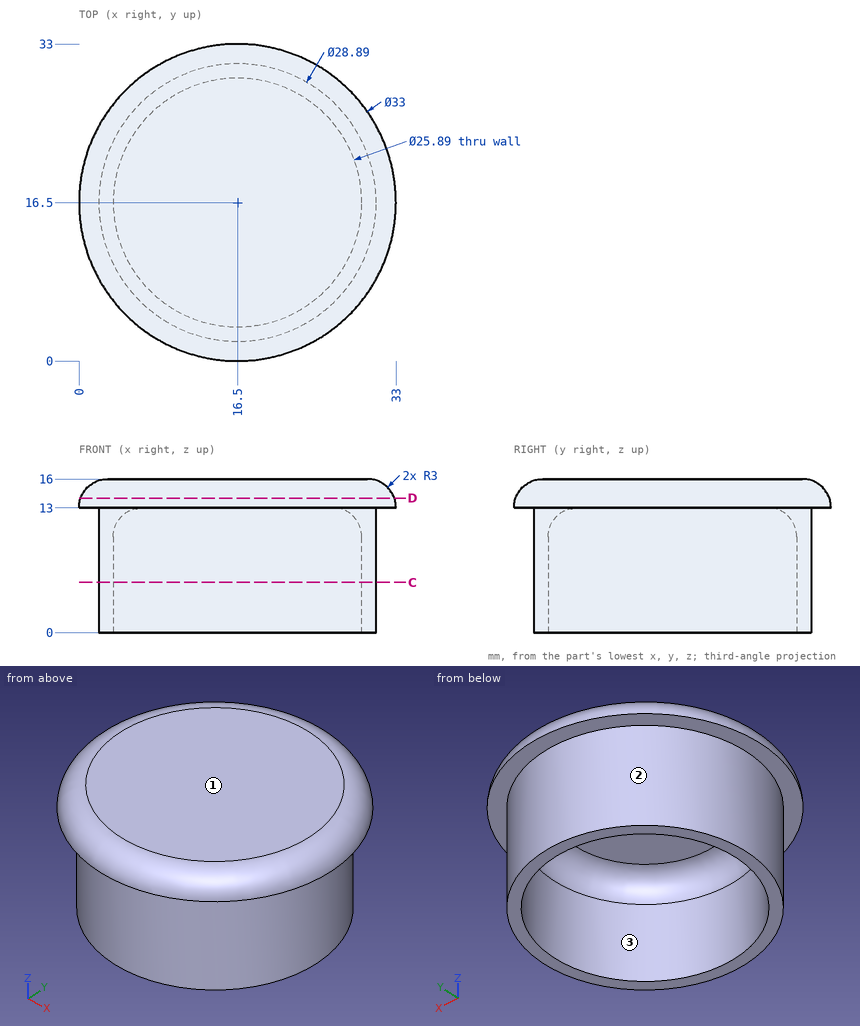
Here's the drawing with two shaded views (mm, measured from the low corner). I have some questions. Round coordinates to 2 decimals unless told otherwise and drop trailing zeros. Write each loop counter-clockwise with the first axis right and the second up, starting at its lowest first coordinate (ties: lowest second). Pieces come first, ordered by that corner, then holes.
(1) If I drill on probe 1 along Y at (x, z) = (16.5, 6) (3 decimals); probe 2 along Z at (x, y) = (18, 17); probe 3 along Y at (x, z) = (5.5, 8.25), over which ranges is the centre line in solid material (lowest first)?
Findings below:
probe 1: y = 2.055 to 3.555, 29.445 to 30.945
probe 2: z = 13 to 16
probe 3: y = 7.14 to 9.68, 23.32 to 25.86
(2) Thinking about a two-plate mould opening in Y: for the marked faces 1, 2 and 3, which applies, +Y half, -Y half, draft (parallel to the pull), parting line (faces both ways), or undercut?
Findings below:
face 1: draft
face 2: parting line
face 3: undercut
(3) Suppose I cut it at D-D on z = 14. Write out the boundary of the cut face in (x, y).
Findings below:
outline: circle Ø32.66 at (16.5, 16.5)
(4) For pin 1 (3 mm diameter, centred on x = 18.5, z = 12.5, fed in from -Y); pin 2 (3 mm diameter, centred on x = 6, z = 13, fed in from +Y); pin 3 (10 mm diameter, centred on x = 20, y = 13, fed in from -Z), each with a flat end and sliding along its axis, tell me the tip position at first contact or that it passes through.
Findings below:
pin 1: stops at y = 0.01
pin 2: stops at y = 30.33
pin 3: stops at z = 13
(5) Suppose I cut it at C-C on z = 5.25. Write out the boundary of the cut face in (x, y) (3 decimals).
Findings below:
outline: circle Ø28.89 at (16.5, 16.5); hole circle Ø25.89 at (16.5, 16.5)
